Source: CAD feature listing. Evaluate the final solid. Frame: model axes, mm. A direction names the side the tool comes from. Round coordinates to 2 decimals unless told otherwise and drop trailing zeros. Order: outer loops, then holes, each group sorted by start corner. A loop starts at its lowest first (then second) coordinate and runs counter-clockwise, first axis right, second up. Notation, with made-up numbers: (15, -32.5) - (48, -32.5) arc R34 ccw to (48, 2.5) - close; hole circle Ø6 at (-11, -21.5). An arc over 180 degrees is marked (long way). Use one line per item in the form item = value. Start each with the question number.
Q1. Cut plane C-C, the plane y = 0.75. Return the cut outline in (x, z), and give its area (3 significant figures).
Q2. Ray query, line 1 (Z direction, x = 140, y = -4.5); line 2 (Z direction, x = 0, y = -5.75); line 3 (X direction, y = 4, z = -6). Return the intervals inside material, ascending. Write a range as [from, to].
Q3. Cut plane A-A, the plane z = 0. Give the number of separate pieces and of enclosed holes in the cut face, and give its area (3 significant figures).
Q4. Pin query (flat end, axial travel): pin 1 Ø6 at (x, z) = (111.48, 0) entering from -Y; pin 2 Ø8 at (x, y) = (32.5, -7) entering from -Z; pin 3 Ø8 at (y, z) = (0, 2) entering from -X; pin 4 Ø1 at (x, y) = (88.5, -3) entering from +Z. Return the tip coordinate at first contact, or that it passes through.
Q5. Set-up query: faces 1 (the flat face through (80.387, 0.14, 17.025)), 2 (the cylindrical face through (127.1, -0.14, -10.07)), 3 (the flat face through (52.829, 0, 0)). Return all of +Z, -Z, +X, -X, +Y, -Y with unobstructed straight access to the full face (end or side cutting, diameter ignored); none if empty.
Q6. Cut plane B-B, the plane x = 0. Return the cut outline in (y, z).
Q7. Draft query along Z for faces 4 (the flat face through (52, -10, -3)), 5 (the flat face through (122.478, 0, 0)), 6 (the flat face through (100.478, 0, 0)), 7 (the cylindrical face through (155, 0, 0)). Return one class per face: released by +Z, released by -Z, zero draft, split by the parting line, or undercut.
Q8. Cut plane D-D, the plane x = 93.5. Return the cut outline in (y, z).
from build123d import *

# Parameters (mm, degrees)
SKETCH1_R           = 30
SKETCH1_R_2         = 7
BOSS_EXTRUDE1_DEPTH = 10
FILLET1_R           = 30
FILLET2_R           = 10
CUT_EXTRUDE1_DEPTH  = 21
BOSS_EXTRUDE2_DEPTH = 20
SKETCH4_R           = 3.5
SKETCH4_R_2         = 5
CUT_EXTRUDE2_DEPTH  = 21


with BuildPart() as part:
    # Sketch1 → Boss-Extrude1 (new body, symmetric)
    with BuildSketch(Plane(origin=(0, 0, 0), x_dir=(1, 0, 0), z_dir=(0, 1, 0))):
        with BuildLine():
            Line((27.935473676, 25.760615491), (128.063755469, 9.084385863))
            ThreePointArc((128.063755469, 9.084385863), (155, 0), (128.063755469, -9.084385863))
            Line((128.063755469, -9.084385863), (27.935473676, -25.760615491))
            ThreePointArc((27.935473676, -25.760615491), (-38, 0), (27.935473676, 25.760615491))
        make_face()
        Circle(SKETCH1_R, mode=Mode.SUBTRACT)
        with Locations((140, 0)):
            Circle(SKETCH1_R_2, mode=Mode.SUBTRACT)
    extrude(amount=BOSS_EXTRUDE1_DEPTH, both=True)

    # Fillet1
    fillet1_edges = [part.edges().sort_by_distance(p)[0] for p in [
        (27.935473676, 0, 25.760615491),
        (27.935473676, 0, -25.760615491),
    ]]
    fillet(fillet1_edges, radius=FILLET1_R)

    # Fillet2
    fillet2_edges = [part.edges().sort_by_distance(p)[0] for p in [
        (128.063755469, 0, 9.084385863),
        (128.063755469, 0, -9.084385863),
    ]]
    fillet(fillet2_edges, radius=FILLET2_R)

    # Sketch2 → Cut-Extrude1 (cut, through all)
    with BuildSketch(Plane(origin=(0, 10, 0), x_dir=(1, 0, 0), z_dir=(0, 1, 0))):
        with BuildLine():
            Line((41.828554558, 17.870982725), (122.478416149, 4.438857582))
            ThreePointArc((122.478416149, 4.438857582), (126.239130435, 0), (122.478416149, -4.438857582))
            Line((122.478416149, -4.438857582), (41.828554558, -17.870982725))
            ThreePointArc((41.828554558, -17.870982725), (37.231968897, -16.217361812), (36.238855523, -11.43439331))
            ThreePointArc((36.238855523, -11.43439331), (38, 0), (36.238855523, 11.43439331))
            ThreePointArc((36.238855523, 11.43439331), (37.231968897, 16.217361812), (41.828554558, 17.870982725))
        make_face()
    extrude(amount=-CUT_EXTRUDE1_DEPTH, mode=Mode.SUBTRACT)

    # Sketch3 → Boss-Extrude2 (add)
    with BuildSketch(Plane(origin=(0, 10, 0), x_dir=(1, 0, 0), z_dir=(0, 1, 0))):
        Polygon((100.478416149, 8.102927765), (122.478416149, 4.438857582), (122.478416149, -4.438857582), (100.478416149, -8.102927765), align=None)
        Polygon((41.828554558, 17.870982725), (52.828554558, 16.038947633), (52.828554558, -16.038947633), (41.828554558, -17.870982725), align=None)
    extrude(amount=-BOSS_EXTRUDE2_DEPTH)

    # Sketch4 → Cut-Extrude2 (cut, through all)
    with BuildSketch(Plane(origin=(0, 10, 0), x_dir=(1, 0, 0), z_dir=(0, 1, 0))):
        with Locations((47.328554558, 0)):
            Circle(SKETCH4_R)
        with Locations((111.478416149, 0)):
            Circle(SKETCH4_R_2)
    extrude(amount=-CUT_EXTRUDE2_DEPTH, mode=Mode.SUBTRACT)


solid = part.part
Completed:
q1.outline = (23.15, -30.14) arc R30 cw to (36.49, -24.34) - (123.07, -9.92) arc R10 cw to (130.83, -11.87) arc R15 ccw (long way) to (130.83, 11.87) arc R10 cw to (123.07, 9.92) - (36.49, 24.34) arc R30 cw to (23.15, 30.14) arc R38 ccw (long way) to start; hole circle Ø60 at (0, 0); hole (36.24, -11.43) arc R5 ccw to (41.83, -17.87) - (41.83, 17.87) arc R5 ccw to (36.24, 11.43) arc R38 cw to start; hole circle Ø7 at (47.33, 0); hole (52.83, -16.04) - (100.48, -8.1) - (100.48, 8.1) - (52.83, 16.04) - close; hole circle Ø10 at (111.48, 0); hole (122.48, -4.44) arc R4.5 ccw to (122.48, 4.44) - close; hole circle Ø14 at (140, 0)
q1.area = 3,920 mm2
q2.line_1 = [-15, -7], [7, 15]
q2.line_2 = [-38, -30], [30, 38]
q2.line_3 = [-37.52, -29.39], [29.39, 37.52], [41.83, 52.83], [100.48, 136.39], [143.61, 153.75]
q3.separate_pieces = 8
q3.enclosed_holes = 0
q3.area = 935 mm2
q4.pin_1 = through
q4.pin_2 = -26.85
q4.pin_3 = -38
q4.pin_4 = 15.76
q5.face_1 = +Z, +Y, -Y
q5.face_2 = -Z, +Y, -Y
q5.face_3 = +Y, -Y
q6.outline = (-10, -38) - (10, -38) - (10, -30) - (-10, -30) - close; (-10, 30) - (10, 30) - (10, 38) - (-10, 38) - close
q7.face_4 = zero draft
q7.face_5 = undercut
q7.face_6 = undercut
q7.face_7 = split by the parting line
q8.outline = (-10, -14.84) - (10, -14.84) - (10, -9.27) - (-10, -9.27) - close; (-10, 9.27) - (10, 9.27) - (10, 14.84) - (-10, 14.84) - close
